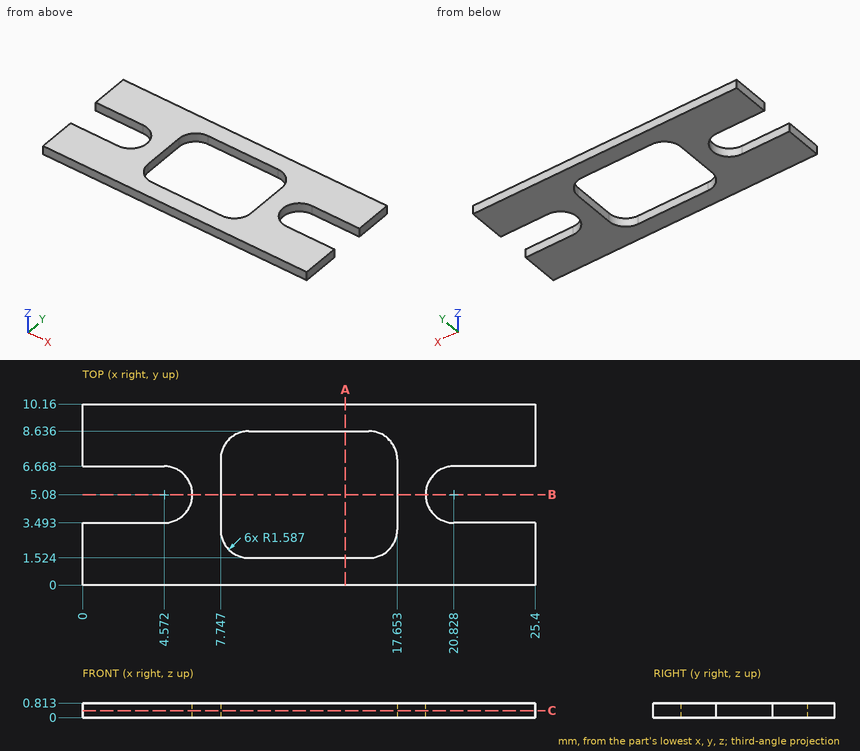
Design review of the part shown in the three views and the two pictorial views. Dimensions are in mm from the part's minimum x, y and z. Round coordinates to 2 decimals unless told otherwise and drop trailing zeros. Write each loop counter-clockwise with the first axis right and the second up, starting at its lowest first coordinate (ties: lowest second). Pieces come first, ordered by that corner, then holes. Notation, with made-up numbers: (57, 33.5) -> (88, 33.5) arc R31 ccw to (88, 60.5) -> close; hole circle Ø2 at (0.25, 25.25). An arc over 180 degrees is marked (long way). Answer as a JSON object with one key per item and string values.
1. Clearance check with flat-ended pins moving along their axes: pin 1 (2 mm diameter, centred on x = 8.5, y = 6, fed in from -Z); pin 2 (3 mm diameter, centred on x = 12.5, y = 6.5, fed in from +Z). State where each tip first meets the part, or that it passes through.
Results found:
{"pin 1": "stops at z = 0", "pin 2": "passes through"}
2. We need section B-B on y = 5.08. State the section outline as (x, z) points.
Results found:
{"outline": "(6.16, 0) -> (7.75, 0) -> (7.75, 0.81) -> (6.16, 0.81) -> close; (17.65, 0) -> (19.24, 0) -> (19.24, 0.81) -> (17.65, 0.81) -> close"}
3. To check wall thickness, follow line 1 along Y through (x, z) = (2.25, 0.2); line 2 along X through (y, z) = (6.75, 0.35); line 3 along Y through (x, z) = (14.5, 0.2) (1 decimal). State the ranges of each line that lie inside material, in increasing order.
Results found:
{"line 1": "y = 0 to 3.49, 6.67 to 10.16", "line 2": "x = 0 to 7.75, 17.65 to 25.4", "line 3": "y = 0 to 1.5, 8.6 to 10.2"}
4. We need section C-C on z = 0.4. State the section outline as (x, y) points (1 decimal).
Results found:
{"outline": "(0, 0) -> (25.4, 0) -> (25.4, 3.5) -> (20.8, 3.5) arc R1.6 cw to (20.8, 6.7) -> (25.4, 6.7) -> (25.4, 10.2) -> (0, 10.2) -> (0, 6.7) -> (4.6, 6.7) arc R1.6 cw to (4.6, 3.5) -> (0, 3.5) -> close; hole (7.7, 3.1) arc R1.6 ccw to (9.3, 1.5) -> (16.1, 1.5) arc R1.6 ccw to (17.7, 3.1) -> (17.7, 7) arc R1.6 ccw to (16.1, 8.6) -> (9.3, 8.6) arc R1.6 ccw to (7.7, 7) -> close"}
5. We need section A-A on x = 14.75. State the section outline as (y, z) points (1 decimal).
Results found:
{"outline": "(0, 0) -> (1.5, 0) -> (1.5, 0.8) -> (0, 0.8) -> close; (8.6, 0) -> (10.2, 0) -> (10.2, 0.8) -> (8.6, 0.8) -> close"}
